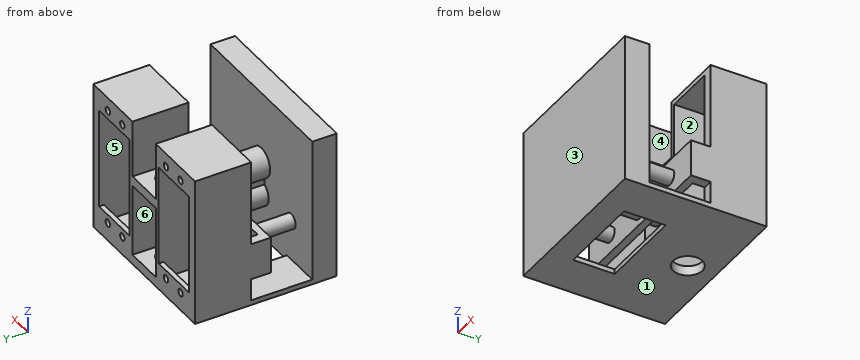
```python
from build123d import *

# Parameters (mm, degrees)
EXTRUDE_1_DEPTH     = 23
EXTRUDE_1_2_DEPTH   = 23
SKETCH_2_W          = 21
SKETCH_2_H          = 9
EXTRUDE_2_DEPTH     = 2
SKETCH_3_R          = 1.5
CUT_EXTRUDE_1_DEPTH = 2
SKETCH_4_W          = 4.5
SKETCH_4_H          = 23
EXTRUDE_3_DEPTH     = 20
SKETCH_5_W          = 20
SKETCH_5_H          = 23
EXTRUDE_4_DEPTH     = 54.5
SKETCH_7_R          = 6
EXTRUDE_5_DEPTH     = 35
SKETCH_8_W          = 4
SKETCH_8_H          = 15
EXTRUDE_6_DEPTH     = 5
EXTRUDE_7_DEPTH     = 3
SKETCH_10_R         = 5
EXTRUDE_8_DEPTH     = 35
EXTRUDE_9_DEPTH     = 35
SKETCH_12_R         = 3
EXTRUDE_10_DEPTH    = 27
CUT_EXTRUDE_2_DEPTH = 27
CUT_EXTRUDE_3_DEPTH = 20
EXTRUDE_11_DEPTH    = 2
SKETCH_16_W         = 35
SKETCH_16_H         = 27
CUT_EXTRUDE_5_DEPTH = 2
SKETCH_18_W         = 16
SKETCH_18_H         = 2
CUT_EXTRUDE_7_DEPTH = 30
SKETCH_19_R         = 3
CUT_EXTRUDE_8_DEPTH = 50
EXTRUDE_12_DEPTH    = 10
SKETCH_21_R         = 6
CUT_EXTRUDE_9_DEPTH = 60


with BuildPart() as part:
    # Sketch 1 → Extrude 1 (new body)
    with BuildSketch(Plane(origin=(0, 0, 0), x_dir=(1, 0, 0), z_dir=(0, 1, 0))):
        Polygon((-66, 57), (-45, 57), (-45, 59), (-70, 59), (-70, 0), (-45, 0), (-45, 2), (-66, 2), align=None)
    extrude(amount=EXTRUDE_1_DEPTH)



with BuildPart() as body_2:
    # Sketch 1 → Extrude 1 2 (new body)
    with BuildSketch(Plane(origin=(0, 0, 0), x_dir=(1, 0, 0), z_dir=(0, 1, 0))):
        Polygon((-25, 2), (-4, 2), (-4, 57), (-25, 57), (-25, 59), (0, 59), (0, 0), (-25, 0), align=None)
    extrude(amount=EXTRUDE_1_2_DEPTH)


with BuildPart() as part_1:
    add(part.part)

    add(body_2.part)  # Extrude 2 merges body 2
    # Sketch 2 → Extrude 2 (add)
    with BuildSketch(Plane(origin=(0, 23, 0), x_dir=(1, 0, 0), z_dir=(0, 1, 0))):
        with Locations((-55.5, 54.5)):
            Rectangle(SKETCH_2_W, SKETCH_2_H)
        with Locations((-14.5, 54.5)):
            Rectangle(SKETCH_2_W, SKETCH_2_H)
        with Locations((-55.5, 4.5)):
            Rectangle(SKETCH_2_W, SKETCH_2_H)
        with Locations((-14.5, 4.5)):
            Rectangle(SKETCH_2_W, SKETCH_2_H)
    extrude(amount=-EXTRUDE_2_DEPTH)

    # Sketch 3 → Cut-Extrude 1 (cut)
    with BuildSketch(Plane(origin=(0, 23, 0), x_dir=(1, 0, 0), z_dir=(0, 1, 0))):
        with Locations((-50, 53.5)):
            Circle(SKETCH_3_R)
        with Locations((-60, 53.5)):
            Circle(SKETCH_3_R)
        with Locations((-20, 53.5)):
            Circle(SKETCH_3_R)
        with Locations((-10, 53.5)):
            Circle(SKETCH_3_R)
        with Locations((-60, 5.5)):
            Circle(SKETCH_3_R)
        with Locations((-50, 5.5)):
            Circle(SKETCH_3_R)
        with Locations((-20, 5.5)):
            Circle(SKETCH_3_R)
        with Locations((-10, 5.5)):
            Circle(SKETCH_3_R)
    extrude(amount=-CUT_EXTRUDE_1_DEPTH, mode=Mode.SUBTRACT)

    # Sketch 4 → Extrude 3 (add)
    with BuildSketch(Plane.ZY.offset(25)):
        with Locations((-56.75, 11.5)):
            Rectangle(SKETCH_4_W, SKETCH_4_H)
    extrude(amount=EXTRUDE_3_DEPTH)

    # Sketch 5 → Extrude 4 (add)
    with BuildSketch(Plane.XY.offset(-54.5)):
        with Locations((-35, 11.5)):
            Rectangle(SKETCH_5_W, SKETCH_5_H)
    extrude(amount=EXTRUDE_4_DEPTH)

    # Sketch 7 → Extrude 5 (add)
    with BuildSketch(Plane.XZ):
        with Locations((-35, -29.5)):
            Circle(SKETCH_7_R)
    extrude(amount=EXTRUDE_5_DEPTH)

    # Sketch 8 → Extrude 6 (add)
    with BuildSketch(Plane.XZ):
        with Locations((-2, -42.5)):
            Rectangle(SKETCH_8_W, SKETCH_8_H)
        with Locations((-68, -42.5)):
            Rectangle(SKETCH_8_W, SKETCH_8_H)
    extrude(amount=EXTRUDE_6_DEPTH)

    # Sketch 9 → Extrude 7 (add)
    with BuildSketch(Plane.XZ.offset(5)):
        Polygon((-70, -50), (-45, -50), (0, -50), (0, -35), (-70, -35), align=None)
    extrude(amount=EXTRUDE_7_DEPTH)

    # Sketch 10 → Extrude 8 (add)
    with BuildSketch(Plane.XZ):
        with Locations((-35, -42.5)):
            Circle(SKETCH_10_R)
    extrude(amount=EXTRUDE_8_DEPTH)

    # Sketch 11 → Extrude 9 (add)
    with BuildSketch(Plane.XZ.offset(35)):
        Polygon((-35, -29.5), (-33, -29.5), (-33, -42.5), (-37, -42.5), (-37, -29.5), align=None)
    extrude(amount=-EXTRUDE_9_DEPTH)

    # Sketch 12 → Extrude 10 (add)
    with BuildSketch(Plane.XZ.offset(8)):
        with Locations((-55.5, -42.5)):
            Circle(SKETCH_12_R)
        with Locations((-14.5, -42.5)):
            Circle(SKETCH_12_R)
    extrude(amount=EXTRUDE_10_DEPTH)

    # Sketch 13 → Cut-Extrude 2 (cut)
    with BuildSketch(Plane.XZ):
        Polygon((-35, -23.5), (-27, -23.5), (-27, -2), (-43, -2), (-43, -23.5), align=None)
    extrude(amount=-CUT_EXTRUDE_2_DEPTH, mode=Mode.SUBTRACT)

    # Sketch 14 → Cut-Extrude 3 (cut)
    with BuildSketch(Plane(origin=(0, 23, 0), x_dir=(1, 0, 0), z_dir=(0, 1, 0))):
        Polygon((-27, 57), (-35, 57), (-43, 57), (-43, 27.5), (-35, 27.5), (-27, 27.5), align=None)
    extrude(amount=-CUT_EXTRUDE_3_DEPTH, mode=Mode.SUBTRACT)

    # Sketch 15 → Extrude 11 (add)
    with BuildSketch(Plane(origin=(0, 0, -59), x_dir=(-1, 0, 0), z_dir=(0, 0, -1))):
        Polygon((0, 0), (0, 23), (70, 23), (70, -35), (0, -35), align=None)
    extrude(amount=EXTRUDE_11_DEPTH)

    # Sketch 16 → Cut-Extrude 5 (cut)
    with BuildSketch(Plane.XY.offset(-59)):
        with Locations((-35, -21.5)):
            Rectangle(SKETCH_16_W, SKETCH_16_H)
    extrude(amount=-CUT_EXTRUDE_5_DEPTH, mode=Mode.SUBTRACT)

    # Sketch 18 → Cut-Extrude 7 (cut)
    with BuildSketch(Plane(origin=(0, 23, 0), x_dir=(1, 0, 0), z_dir=(0, 1, 0))):
        with Locations((-35, 1)):
            Rectangle(SKETCH_18_W, SKETCH_18_H)
    extrude(amount=-CUT_EXTRUDE_7_DEPTH, mode=Mode.SUBTRACT)

    # Sketch 19 → Cut-Extrude 8 (cut)
    with BuildSketch(Plane.XY.offset(-23.5)):
        with Locations((-35, 11.5)):
            Circle(SKETCH_19_R)
    extrude(amount=-CUT_EXTRUDE_8_DEPTH, mode=Mode.SUBTRACT)

    # Sketch 20 → Extrude 12 (add)
    with BuildSketch(Plane.XZ.offset(35)):
        Polygon((-35, 0), (0, 0), (0, -61), (-70, -61), (-70, 0), align=None)
    extrude(amount=-EXTRUDE_12_DEPTH)

    # Sketch 21 → Cut-Extrude 9 (cut)
    with BuildSketch(Plane.XY.offset(-23.5)):
        with Locations((-35, 11.5)):
            Circle(SKETCH_21_R)
    extrude(amount=-CUT_EXTRUDE_9_DEPTH, mode=Mode.SUBTRACT)


solid = part_1.part
```
Part model, mm, in its own coordinate system. Face numbers are marked on the shaded views. A direction names the side the tool comes from. Round coordinates to 2 decimals unless told otherwise and drop trailing zeros. Write each loop counter-clockwise with the first axis right and the second up, starting at its lowest first coordinate (ties: lowest second). Pieces come first, ordered by that corner, then holes. Notation, with made-up numbers: M 40,34.5 L 91,34.5 A28 ccw 91,66.5 Z; hole C 64,49 d2. An arc over 180 degrees is marked long. Answer as CSV lines item,"result". Start each with the question number.
1) Band-saw the part on B-B (x = -10). List the corners of the cut face in (y, z).
2) Drill centre lines: L1, parallel to X at y = 5, z = -20.5; L2, parallel to Y at x = -35, z = -58.3; L3, parallel to Z at x = -50, y = 22.4. Where is each one in solid material? Low to high.
3) Band-saw the part on D-D (z = -25). List the corners of the cut face in (x, y), then the cut area to 3 significant figures.
4) Drop flat-ended pins along their axis: pin 1 (5 mm diameter, centred on x = -31.5, y = 17, fed in from +Z); pin 2 (2 mm diameter, centred on x = -51, z = -27.5, fed in from +Y); pin 3 (8 mm diameter, centred on x = -34, z = -38, fed in from +Y). Give the stop position or say it passes through.
5) Mould opens along Z. For the marked faces 1, 2 and 3 say: +Z half, -Z half, draft (parallel to the pull), parting line (faces both ways), or undercut.
6) Which spindle directions (+Z, -Z, +X, -X, +Y, -Y) get a long thin tool onto all of the face, cutting with end or side? Do the marked faces 4, 5 and 6. Say none if no direction does.
7) Band-saw the part on C-C (y = -10.5). List the corners of the cut face in (x, z), then the cut area to 3 significant figures.
8) Band-saw the part on A-A (y = 11.5). List the corners of the cut face in (x, z), then the cut area to 3 significant figures.
Worked out:
1,outline,"M -35,-61 L 23,-61 L 23,-55 L 21,-55 L 21,-57 L 0,-57 L 0,-59 L -25,-59 L -25,0 L -35,0 Z; M -8,-50 L -5,-50 L -5,-35 L -8,-35 Z; M 0,-2 L 21,-2 L 21,-4 L 23,-4 L 23,0 L 0,0 Z; M 21,-52 L 23,-52 L 23,-50 L 21,-50 Z; M 21,-9 L 23,-9 L 23,-7 L 21,-7 Z"
2,L1,"-70 to -66, -45 to -43, -27 to -25, -4 to 0"
2,L2,"-35 to -25, 0 to 5.5, 17.5 to 23"
2,L3,"-61 to -55, -52 to -50, -9 to -7, -4 to 0"
3,outline,"M -70,-35 L 0,-35 L 0,-25 L -31.03,-25 L -31.03,0 L -25,0 L -25,23 L -45,23 L -45,0 L -38.97,0 L -38.97,-25 L -70,-25 Z; M -70,0 L -66,0 L -66,23 L -70,23 Z; M -4,0 L 0,0 L 0,23 L -4,23 Z; hole C -35,11.5 d12"
3,area,"1,430 mm²"
4,pin 1,"z = -23.5"
4,pin 2,"y = -25"
4,pin 3,"y = 3"
5,face 1,"-Z half"
5,face 2,"undercut"
5,face 3,"draft"
6,face 4,"+Z, +Y"
6,face 5,"none"
6,face 6,"+Y"
7,outline,"M -70,-61 L -52.5,-61 L -52.5,-59 L -70,-59 Z; C -55.5,-42.5 d6; M -37,-37.92 A5 ccw long -33,-37.92 L -33,-35.16 A6 ccw long -37,-35.16 Z; M -17.5,-61 L 0,-61 L 0,-59 L -17.5,-59 Z; C -14.5,-42.5 d6"
7,area,"327 mm²"
8,outline,"M -70,-61 L -41,-61 L -41,-57 L -43,-57 L -43,-27.5 L -41,-27.5 L -41,-23.5 L -43,-23.5 L -43,0 L -70,0 Z; M -29,-61 L 0,-61 L 0,0 L -27,0 L -27,-23.5 L -29,-23.5 L -29,-27.5 L -27,-27.5 L -27,-57 L -29,-57 Z; hole M -66,-57 L -45,-57 L -45,-2 L -66,-2 Z; hole M -25,-57 L -4,-57 L -4,-2 L -25,-2 Z"
8,area,"1,020 mm²"
